Can you work these out from the model? Positions are in its coordinate system, mm. A direction names the side the tool comes from. Round coordinates to 2 decimals unless told otherwise and drop trailing zeros. Write each loop counter-clockwise with the first axis right and the second up, starting at its lowest first coordinate (ties: lowest second). Pieces come first, ordered by that corner, then holes.
Q1. For faces 1 (the flat face through (16.5, -12, 1)), 2 (the flat face through (16.5, 9, 1)), 3 (the flat face through (-8, -13.5, 1)), 4 (the flat face through (16.5, 34, 1)), which set-ups out of +Z, -Z, +X, -X, +Y, -Y let a thin tool reach every point of the face, with its end or its side?
Q2. If we section it at A-A (z = 1.35): Please give me the cut outline in (x, y), plus the area to 3 significant figures.
Q3. If we section it at D-D (y = 0): Please give me the cut outline in (x, z).
Q4. I'm going to push flat-ended pins straight in: pin 1 Ø0.8 at (x, z) = (17, 1.5) entering from +Y; pin 2 Ø6 at (x, y) = (0.5, 24.5) entering from +Z; pin 3 Ø1.5 at (y, z) = (34, 2) entering from +X. Where does each tip first touch, or does it pass through?
Q5. If we section it at C-C (y = 27): Please give me the cut outline in (x, z), plus the area to 3 significant figures.
Q6. We'd pull the mould along Y, two halves only. Please class faces 5 (the cylindrical face through (8.5, 27.1, 1.5)), 6 (the flat face through (19, 19, 1)), 7 (the flat face through (0, 37.65, 1)), 8 (the flat face through (16, 23, 1)): +Y half, -Y half, draft (parallel to the pull), parting line (faces both ways), or undercut.
Q7. Please list where these lines run through material, in increasing order: line 1 along Y through (x, z) = (-13, 1.8); line 2 along Y through (x, z) = (11.5, 2.45); line 3 along Y through (x, z) = (14, 0.5).
Q8. If we section it at B-B (x = 10.5): Please give me the cut outline in (y, z).
from build123d import *

# Parameters (mm, degrees)
BOSS_EXTRU_1_DEPTH = 3


with BuildPart() as part:
    # Esquisse1 → Boss.-Extru.1 (new body)
    with BuildSketch(Plane.XY):
        with BuildLine():
            Line((-16, 33.65), (-16, 37.65))
            Line((-16, 37.65), (16.5, 37.65))
            Line((16.5, 37.65), (16.5, 31))
            Line((16.5, 31), (12.5, 31))
            ThreePointArc((12.5, 31), (8.5, 27), (12.5, 23))
            Line((12.5, 23), (19, 23))
            Line((19, 23), (19, 15))
            Line((19, 15), (16.5, 15))
            Line((16.5, 15), (16.5, 2))
            Line((16.5, 2), (19, 2))
            Line((19, 2), (19, -6))
            Line((19, -6), (16.5, -6))
            Line((16.5, -6), (16.5, -17.5))
            Line((16.5, -17.5), (-16, -17.5))
            Line((-16, -17.5), (-16, -13.5))
            Line((-16, -13.5), (0, -13.5))
            ThreePointArc((0, -13.5), (13.5, 0), (0, 13.5))
            Line((0, 13.5), (-16, 13.5))
            Line((-16, 13.5), (-16, 20.35))
            Line((-16, 20.35), (1.5, 20.35))
            Line((1.5, 20.35), (1.5, 33.65))
            Line((1.5, 33.65), (-16, 33.65))
        make_face()
    extrude(amount=BOSS_EXTRU_1_DEPTH)


solid = part.part
A:
1. face 1: +Z, -Z, +X, -Y
1. face 2: +Z, -Z, +X
1. face 3: +Z, -Z, -X
1. face 4: +Z, -Z, +X, +Y
2. outline: (-16, -17.5) - (16.5, -17.5) - (16.5, -6) - (19, -6) - (19, 2) - (16.5, 2) - (16.5, 15) - (19, 15) - (19, 23) - (12.5, 23) arc R4 cw to (12.5, 31) - (16.5, 31) - (16.5, 37.65) - (-16, 37.65) - (-16, 33.65) - (1.5, 33.65) - (1.5, 20.35) - (-16, 20.35) - (-16, 13.5) - (0, 13.5) arc R13.5 cw to (0, -13.5) - (-16, -13.5) - close
2. area: 824 mm2
3. outline: (13.5, 0) - (19, 0) - (19, 3) - (13.5, 3) - close
4. pin 1: stops at y = 23
4. pin 2: stops at z = 3
4. pin 3: stops at x = 16.5
5. outline: (1.5, 0) - (8.5, 0) - (8.5, 3) - (1.5, 3) - close
5. area: 21.0 mm2
6. face 5: undercut
6. face 6: draft
6. face 7: +Y half
6. face 8: undercut
7. line 1: y = -17.5 to -13.5, 13.5 to 20.35, 33.65 to 37.65
7. line 2: y = -17.5 to -7.07, 7.07 to 23.13, 30.87 to 37.65
7. line 3: y = -17.5 to 23, 31 to 37.65
8. outline: (-17.5, 0) - (-8.49, 0) - (-8.49, 3) - (-17.5, 3) - close; (8.49, 0) - (23.54, 0) - (23.54, 3) - (8.49, 3) - close; (30.46, 0) - (37.65, 0) - (37.65, 3) - (30.46, 3) - close
